The drawing under review shows one solid part. Ordinate dimensions are in mm from its lowest x, y, z. Round coordinates to 2 decimals unless told otherwise and drop trailing zeros. Order: outer loops, then holes, each group sorted by start corner. A loop starts at its lowest first (then second) coordinate and runs counter-clockwise, first axis right, second up. Notation, with made-up numbers: M -8.5,32.5 L 40.5,32.5 A27 ccw 40.5,67.5 Z; hole C 64,69 d5. An arc over 180 degrees is marked long. Use a Markdown table: item, result.
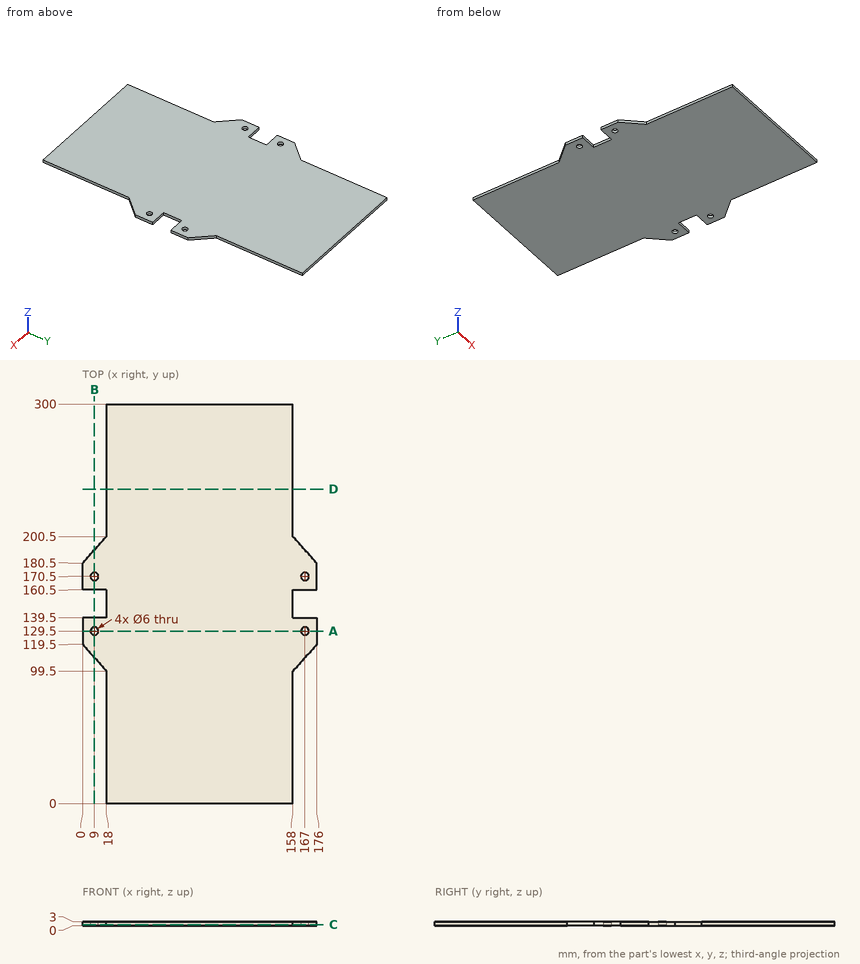
Q1. Add section B-B (x = 9). Write out the cut boundary in (y, z), then the cut area to 3 significant figures.
Determined:
| item | result |
|---|---|
| outline | M 109.5,0 L 126.5,0 L 126.5,3 L 109.5,3 Z; M 132.5,0 L 139.5,0 L 139.5,3 L 132.5,3 Z; M 160.5,0 L 167.5,0 L 167.5,3 L 160.5,3 Z; M 173.5,0 L 190.5,0 L 190.5,3 L 173.5,3 Z |
| area | 144 mm^2 |
Q2. Clearance check with flat-ended pins moving along their axes: pin 1 (0.9 mm diameter, centred on x = 6, z = 1.5, fed in from +Y); pin 2 (0.9 mm diameter, centred on y = 155, z = 1, fed in from -X); pin 3 (5.5 mm diameter, centred on x = 9, y = 170.5, fed in from -Z); pin 4 (1.5 mm diameter, centred on x = 167, z = 1, fed in from -Y). State where each tip first meets the part, or that it passes through.
Determined:
| item | result |
|---|---|
| pin 1 | stops at y = 187.67 |
| pin 2 | stops at x = 18 |
| pin 3 | passes through |
| pin 4 | stops at y = 108.67 |
Q3. Add section D-D (y = 236). Write out the cut boundary in (x, z).
Determined:
| item | result |
|---|---|
| outline | M 18,0 L 158,0 L 158,3 L 18,3 Z |
Q4. Wall thickness on line 1 along X through (y, z) = (170.5, 2.3); line 2 along X through (y, z) = (168, 2.45); line 3 along Y through (x, z) = (9, 1.6): over which ranges is each line inside the solid? List them lowest first. Write a range as [from, to].
Determined:
| item | result |
|---|---|
| line 1 | x = [0, 6], [12, 164], [170, 176] |
| line 2 | x = [0, 7.34], [10.66, 165.34], [168.66, 176] |
| line 3 | y = [109.5, 126.5], [132.5, 139.5], [160.5, 167.5], [173.5, 190.5] |
Q5. Add section C-C (z = 0.75). Write out the cut boundary in (x, y).
Determined:
| item | result |
|---|---|
| outline | M 0,119.5 L 18,99.5 L 18,0 L 158,0 L 158,99.5 L 176,119.5 L 176,139.5 L 158,139.5 L 158,160.5 L 176,160.5 L 176,180.5 L 158,200.5 L 158,300 L 18,300 L 18,200.5 L 0,180.5 L 0,160.5 L 18,160.5 L 18,139.5 L 0,139.5 Z; hole C 9,129.5 d6; hole C 9,170.5 d6; hole C 167,129.5 d6; hole C 167,170.5 d6 |
Q6. Add section A-A (y = 129.5). Write out the cut boundary in (x, z), then the cut area to 3 significant figures.
Determined:
| item | result |
|---|---|
| outline | M 0,0 L 6,0 L 6,3 L 0,3 Z; M 12,0 L 164,0 L 164,3 L 12,3 Z; M 170,0 L 176,0 L 176,3 L 170,3 Z |
| area | 492 mm^2 |
